Read the model definition and answer for the solid it produces. Units are mm, in the model's axes. Face numbers are marked on the shaded views. A direction names the side the tool comes from. Coordinates: 2 decimals unless noted, no trailing zeros. Order: outer loops, then holes, each group sorted by start corner. A loop starts at its lowest first (then second) coordinate and runs counter-clockwise, first axis right, second up. Notation, with made-up numbers: M 51.5,-38.5 L 81.5,-38.5 A16 ccw 81.5,-20.5 Z; hole C 2,-30 d3. An arc over 180 degrees is marked long. Write each question's results on one line, items separated by ' | '.
```python
from build123d import *

# Parameters (mm, degrees)
CHAMFER1_SIZE           = 0.5
CHAMFER2_SIZE           = 0.5
BOSS_EXTRUDE1_START     = -2
SKETCH3_R               = 28.025
BOSS_EXTRUDE1_DEPTH     = 2
CUT_EXTRUDE1_DEPTH      = 54.38539126
CUT_EXTRUDE1_DEPTH_BACK = 54.38539126
SKETCH4_W               = 71.155629785
SKETCH4_H               = 10.339888571
SKETCH5_R               = 31.5
CUT_EXTRUDE2_DEPTH      = 13


with BuildPart() as part:
    # Sketch1 → Revolve1 (revolve)
    with BuildSketch(Plane(origin=(0, 0, 0), x_dir=(1, 0, 0), z_dir=(0, 1, 0)), mode=Mode.PRIVATE) as revolve1_sk:
        Polygon((25.025, 0), (25.025, 20), (28.025, 20), (28.025, 15), (35, 15), (35, 10), (34, 10), (34, 7.5), (33, 7.5), (33, 2.5), (34, 2.5), (34, 0), align=None)
    revolve(revolve1_sk.sketch.rotate(Axis((0, 0, -99.297916667), (0, 0, 1)), 180), axis=Axis((0, 0, -99.297916667), (0, 0, 1)))

    # Chamfer1
    chamfer1_edges = [part.edges().sort_by_distance(p)[0] for p in [
        (28.025, 0, -20),
        (25.025, 0, -20),
    ]]
    chamfer(chamfer1_edges, length=CHAMFER1_SIZE)

    # Chamfer2
    chamfer2_edges = [part.edges().sort_by_distance(p)[0] for p in [
        (34, 0, -7.5),
        (34, 0, 0),
        (34, 0, -2.5),
        (33, 0, -2.5),
        (33, 0, -7.5),
    ]]
    chamfer(chamfer2_edges, length=CHAMFER2_SIZE - 0.0001)  # a hair under: the kernel refuses the full size

    # Sketch3 → Boss-Extrude1 (add)
    with BuildSketch(Plane(origin=(0, 0, -15), x_dir=(-1, 0, 0), z_dir=(0, 0, -1)).offset(BOSS_EXTRUDE1_START)):
        Circle(SKETCH3_R)
    extrude(amount=BOSS_EXTRUDE1_DEPTH)

    # Sketch4 → Cut-Extrude1 (cut, two sides: drawn at the far end of the back side and taken through both)
    with BuildSketch(Plane(origin=(0, 0, 0), x_dir=(1, 0, 0), z_dir=(0, 1, 0)).offset(-CUT_EXTRUDE1_DEPTH_BACK)):
        with Locations((0.577814893, 20.169944286)):
            Rectangle(SKETCH4_W, SKETCH4_H)
    extrude(amount=CUT_EXTRUDE1_DEPTH + CUT_EXTRUDE1_DEPTH_BACK, mode=Mode.SUBTRACT)

    # Sketch5 → Cut-Extrude2 (cut)
    with BuildSketch(Plane.XY):
        Circle(SKETCH5_R)
    extrude(amount=-CUT_EXTRUDE2_DEPTH, mode=Mode.SUBTRACT)


solid = part.part
```
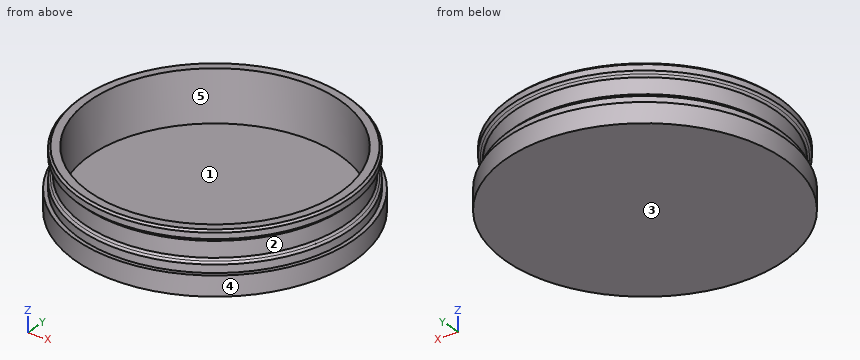
(1) For the marked faces 4 and 5, determine the directions among +Z, -Z, +X, -X, +Y, -Y from which every point of the face is accessible in a straight line to the end or side of a thin tool.
Conclusion:
face 4: +Z, -Z | face 5: +Z
(2) The part is cut by section C-C, the plane z = -4.5. Write down the section's boundary in (x, y), then the cut area to 3 significant figures.
Conclusion:
outline: C 0,0 d66; hole C 0,0 d63 | area: 304 mm²
(3) Straight lines are drawn through the part: line 1 (Y direction, x = 0, z = -8); line 2 (Z direction, x = -13, y = -10); line 3 (Y direction, x = 24, z = -6). For each, find the intervals that lie inside material, in ascending order.
Conclusion:
line 1: -34 to -31.5, 31.5 to 34 | line 2: -15 to -13 | line 3: -22.65 to -20.4, 20.4 to 22.65
(4) Given pin 1 (1 mm diameter, centred on x = 13, z = -2, fed in from -Y); pin 2 (8 mm diameter, centred on x = 2.5, z = -7.5, fed in from +Y); pin 3 (2 mm diameter, centred on x = 20, y = 7, fed in from +Z), each flat-ended and moving along its own axis, determine where each tip first touches the part or whether it passes through.
Conclusion:
pin 1: y = -31.62 | pin 2: y = 35 | pin 3: z = -13
(5) The mould has two halves that part along X. Classify the marked faces 1, 2 and 3: pulls with the +X half, pulls with the -X half, needs draft (parallel to the pull), parting line crosses it, or undercut.
Conclusion:
face 1: undercut | face 2: parting line crosses it | face 3: needs draft
